from build123d import *

# Parameters (mm, degrees)
SKETCH_2_W          = 150
SKETCH_2_H          = 140
EXTRUDE_1_DEPTH     = 140
SKETCH_3_W          = 150
SKETCH_3_H          = 100
CUT_EXTRUDE_1_DEPTH = 110
SKETCH_4_W          = 100
SKETCH_4_H          = 13
CUT_EXTRUDE_2_DEPTH = 231.131739112
SKETCH_5_R          = 3
CUT_EXTRUDE_3_DEPTH = 50
SKETCH_6_R          = 3
CUT_EXTRUDE_4_DEPTH = 177.679477459


with BuildPart() as part:
    # 草圖2 → 填料-伸長1 (new body)
    with BuildSketch(Plane(origin=(0, 0, 0), x_dir=(1, 0, 0), z_dir=(0, 1, 0))):
        with Locations((15.857142857, -34.214285714)):
            Rectangle(SKETCH_2_W, SKETCH_2_H)
    extrude(amount=EXTRUDE_1_DEPTH)

    # 草圖3 → 除料-伸長1 (cut)
    with BuildSketch(Plane(origin=(0, 140, 0), x_dir=(1, 0, 0), z_dir=(0, 1, 0))):
        with Locations((15.857142857, -34.214285714)):
            Rectangle(SKETCH_3_W, SKETCH_3_H)
    extrude(amount=-CUT_EXTRUDE_1_DEPTH, mode=Mode.SUBTRACT)

    # 草圖4 → 除料-伸長2 (cut, through all)
    with BuildSketch(Plane(origin=(90.857142857, 0, 0), x_dir=(0, 0, -1), z_dir=(1, 0, 0))):
        with Locations((-34.214285714, 13.5)):
            Rectangle(SKETCH_4_W, SKETCH_4_H)
    extrude(amount=-CUT_EXTRUDE_2_DEPTH, mode=Mode.SUBTRACT)

    # 草圖5 → 除料-伸長3 (cut)
    with BuildSketch(Plane(origin=(0, 30, 0), x_dir=(1, 0, 0), z_dir=(0, 1, 0))):
        with Locations(Location((70.857142857, -34.214285714, 0), (0, 0, 270))):
            Circle(SKETCH_5_R)
    extrude(amount=-CUT_EXTRUDE_3_DEPTH, mode=Mode.SUBTRACT)

    # 草圖6 → 除料-伸長4 (cut, through all)
    with BuildSketch(Plane(origin=(0, 30, 0), x_dir=(1, 0, 0), z_dir=(0, 1, 0))):
        with Locations(Location((-29.142857143, -34.214285714, 0), (0, 0, 270))):
            Circle(SKETCH_6_R)
    extrude(amount=-CUT_EXTRUDE_4_DEPTH, mode=Mode.SUBTRACT)


solid = part.part
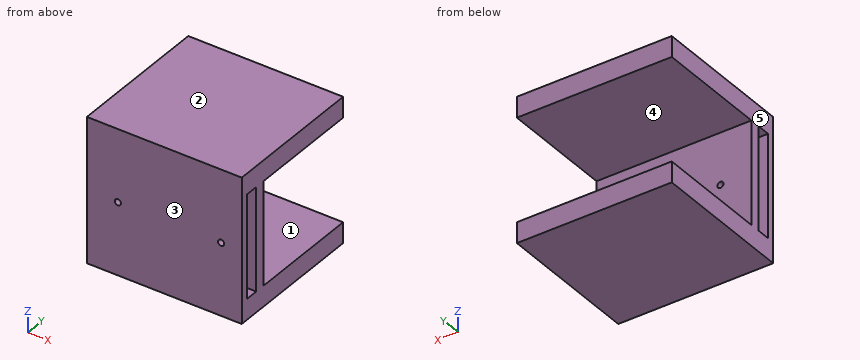
Model file for the job. Use its own axes, mm. Face numbers are marked on the shaded views. A direction names the side the tool comes from. Round coordinates to 2 decimals unless told otherwise and drop trailing zeros. Order: outer loops, then holes, each group sorted by start corner. A loop starts at its lowest first (then second) coordinate and runs counter-clockwise, first axis right, second up.
(1) Band-saw the part on B-B (y = 127.5). List the corners of the cut face in (x, z), then the cut area to 3 significant figures.
(2) Pull direction Z, two halves, no side cores. Call the marked faces 1, 2 and 3: released by +Z, released by -Z, zero draft, split by the parting line, or undercut.
(3) Band-saw the part on C-C (x = -4). List the corners of the cut face in (y, z), then the cut area to 3 significant figures.
(4) Drill centre lines: line 1 (Y direction, x = 46.5, z = 42.5); line 2 (Z direction, x = 9, y = 60.5). Where is each one in solid material? Low to high.
(5) Band-saw the part on A-A (z = -1.5). List the corners of the cut face in (x, y).
(6) 3-axis set-ups, long thin cutter, end or side, ignore diameter. For the marked faces 4 and 5: which of +Z, -Z, +X, -X, +Y, -Y reach the whole face in a straight line?
(7) Pin check, flat tips, straight feed: pin 1 (1 mm diameter, centred on x = 8.5, z = 54.5, fed in from +Y); pin 2 (5 mm diameter, centred on x = -29.14, z = 34.21, fed in from -Y) (3 decimals). Stop position of each tip, or through.
Verdict:
1. outline: (-59.14, -35.79) - (90.86, -35.79) - (90.86, -15.79) - (-59.14, -15.79) - close; (-59.14, 84.21) - (90.86, 84.21) - (90.86, 104.21) - (-59.14, 104.21) - close
1. area: 6,000 mm2
2. face 1: undercut
2. face 2: released by +Z
2. face 3: zero draft
3. outline: (0, -35.79) - (140, -35.79) - (140, -15.79) - (30, -15.79) - (30, 84.21) - (140, 84.21) - (140, 104.21) - (0, 104.21) - close; hole (7, -15.79) - (20, -15.79) - (20, 84.21) - (7, 84.21) - close
3. area: 7,300 mm2
4. line 1: y = 0 to 7, 20 to 30
4. line 2: z = -35.79 to -15.79, 84.21 to 104.21
5. outline: (-59.14, 0) - (90.86, 0) - (90.86, 7) - (-59.14, 7) - close; (-59.14, 20) - (90.86, 20) - (90.86, 30) - (-59.14, 30) - close
6. face 4: +X, -X, +Y
6. face 5: +Z, -Z, -X, +Y, -Y
7. pin 1: stops at y = 30
7. pin 2: passes through
